Design review of the part built by this model. Coordinates are the model's own, in mm. A direction names the side the tool comes from. Round coordinates to 2 decimals unless told otherwise and drop trailing zeros. Write item = value, one per line.
Autodesk Inventor part; units mm, degrees
ref_plane "Start Plane" through (0, 0, 15) normal (0, 0, 1) x (1, 0, 0)
ref_plane "End Plane" through (0, 0, 435) normal (0, 0, 1) x (1, 0, 0)
ref_plane "Work Plane5" through (-185, 5.2, 435) normal (0, 0, 1) x (1, 0, 0)
ref_plane "Work Plane3" through (0, 0, 250) normal (0, 0, 1) x (1, 0, 0)
sketch "Sketch2" plane through (0, 0, 250) normal (0, 0, 1) x (1, 0, 0)
  circle A0 centre (0, 0) radius 3.4
  dimension "d51" = 6.8
extrude "Extrusion2" [suppressed]
ref_plane "Start Plane" through (0, 0, 15) normal (0, 0, 1) x (1, 0, 0)
ref_plane "End Plane" through (0, 0, 435) normal (0, 0, 1) x (1, 0, 0)
sketch "Sketch" plane through (0, 0, 0) normal (0, 0, 1) x (1, 0, 0)
  line L0 (-13, 15) -> (13, 15)
  line L1 (15, 13) -> (15, -13)
  line L2 (-15, 15) -> (15, -15) construction
  line L3 (15, 15) -> (-15, -15) construction
  line L4 (-5.2, 15) -> (-5.2, 14.2)
  line L5 (-5.2, 14.2) -> (-4.1, 14.2)
  line L6 (-4.1, 14.2) -> (-4.1, 12.2)
  line L7 (-4.1, 12.2) -> (-8.25, 12.2)
  line L8 (-8.25, 12.2) -> (-8.25, 10.2)
  line L9 (-8.25, 10.2) -> (-3.85, 5.8)
  line L10 (-3.85, 5.8) -> (3.85, 5.8)
  line L11 (8.25, 12.2) -> (4.1, 12.2)
  line L12 (4.1, 12.2) -> (4.1, 14.2)
  line L13 (4.1, 14.2) -> (5.2, 14.2)
  line L14 (5.2, 14.2) -> (5.2, 15)
  line L15 (8.25, 12.2) -> (8.25, 10.2)
  line L16 (8.25, 10.2) -> (3.85, 5.8)
  line L17 (-5.8, 0) -> (5.8, 0)
  line L18 (-5.2, -15) -> (-5.2, -14.2)
  line L19 (-5.2, -14.2) -> (-4.1, -14.2)
  line L20 (-4.1, -14.2) -> (-4.1, -12.2)
  line L21 (-4.1, -12.2) -> (-8.25, -12.2)
  line L22 (-8.25, -12.2) -> (-8.25, -10.2)
  line L23 (-8.25, -10.2) -> (-3.85, -5.8)
  line L24 (-3.85, -5.8) -> (3.85, -5.8)
  line L25 (8.25, -12.2) -> (4.1, -12.2)
  line L26 (4.1, -12.2) -> (4.1, -14.2)
  line L27 (4.1, -14.2) -> (5.2, -14.2)
  line L28 (5.2, -14.2) -> (5.2, -15)
  line L29 (8.25, -12.2) -> (8.25, -10.2)
  line L30 (8.25, -10.2) -> (3.85, -5.8)
  line L31 (0, 5.8) -> (0, -5.8)
  line L32 (15, 5.2) -> (14.2, 5.2)
  line L33 (14.2, 5.2) -> (14.2, 4.1)
  line L34 (14.2, 4.1) -> (12.2, 4.1)
  line L35 (12.2, 4.1) -> (12.2, 8.25)
  line L36 (15, -5.2) -> (14.2, -5.2)
  line L37 (14.2, -5.2) -> (14.2, -4.1)
  line L38 (14.2, -4.1) -> (12.2, -4.1)
  line L39 (12.2, -4.1) -> (12.2, -8.25)
  line L40 (12.2, -8.25) -> (10.2, -8.25)
  line L41 (10.2, -8.25) -> (5.8, -3.85)
  line L42 (5.8, -3.85) -> (5.8, 3.85)
  line L43 (5.8, 3.85) -> (10.2, 8.25)
  line L44 (10.2, 8.25) -> (12.2, 8.25)
  line L45 (-15, 5.2) -> (-14.2, 5.2)
  line L46 (-14.2, 5.2) -> (-14.2, 4.1)
  line L47 (-14.2, 4.1) -> (-12.2, 4.1)
  line L48 (-12.2, 4.1) -> (-12.2, 8.25)
  line L49 (-15, -5.2) -> (-14.2, -5.2)
  line L50 (-14.2, -5.2) -> (-14.2, -4.1)
  line L51 (-14.2, -4.1) -> (-12.2, -4.1)
  line L52 (-12.2, -4.1) -> (-12.2, -8.25)
  line L53 (-12.2, -8.25) -> (-10.2, -8.25)
  line L54 (-10.2, -8.25) -> (-5.8, -3.85)
  line L55 (-5.8, -3.85) -> (-5.8, 3.85)
  line L56 (-5.8, 3.85) -> (-10.2, 8.25)
  line L57 (-10.2, 8.25) -> (-12.2, 8.25)
  circle A0 centre (11.5, 11.5) radius 1.65
  circle A1 centre (11.5, -11.5) radius 1.65
  circle A2 centre (-11.5, 11.5) radius 1.65
  circle A3 centre (-11.5, -11.5) radius 1.65
  line L58 (-15, -13) -> (-15, -5.2)
  line L59 (-15, 5.2) -> (-15, 13)
  line L60 (13, -15) -> (5.2, -15)
  line L61 (-5.2, -15) -> (-13, -15)
  arc A4 (-13, 15) -> (-15, 13) centre (-13, 13) ccw
  arc A5 (15, 13) -> (13, 15) centre (13, 13) ccw
  arc A6 (13, -15) -> (15, -13) centre (13, -13) ccw
  arc A7 (-15, -13) -> (-13, -15) centre (-13, -13) ccw
  point P0 (0, 0)
  point P1 (0, 0)
  dimension "d2" = 8.2
  dimension "d3" = 4.1
  dimension "d4" = 10.4
  dimension "d5" = 5.2
  dimension "d8" = 9.2
  dimension "d11" = 16.5
  dimension "d12" = 8.25
  dimension "d14" = 0.8
  dimension "d15" = 2
  dimension "d16" = 2
  dimension "d34" = 0.8
  dimension "d35" = 10.4
  dimension "d36" = 5.2
  dimension "d37" = 8.2
  dimension "d38" = 4.1
  dimension "d39" = 2
  dimension "d40" = 16.5
  dimension "d41" = 8.25
  dimension "d42" = 2
  dimension "d43" = 9.2
  dimension "d44" = 23
  dimension "d45" = 11.5
  dimension "d46" = 23
  dimension "d47" = 11.5
  dimension "d48" = 3.3
  dimension "d55" = 2
extrude "Body" add sketch "Sketch" along normal up to surface (420 mm away) from surface at 15 contours L0 L4 L5 L6 L7 L8 L9 L10 L31 L17 L55 L56 L57 L48 L47 L46 L45 L59 A4 | L0 A5 L1 L32 L33 L34 L35 L44 L43 L42 L17 L31 L10 L16 L15 L11 L12 L13 L14 | L1 A6 L60 L28 L27 L26 L25 L29 L30 L24 L31 L17 L42 L41 L40 L39 L38 L37 L36 | L31 L24 L23 L22 L21 L20 L19 L18 L61 A7 L58 L49 L50 L51 L52 L53 L54 L55 L17
sketch "Sketch3" plane through (0, 0, 0) normal (0, 0, 1) x (1, 0, 0)
  line L0 (0, 0) -> (10, 0)
ref_plane "Work Plane4" through (0, 0, 0) normal (0, -1, 0) x (1, 0, 0)
sketch "Sketch4" plane through (0, 0, 0) normal (0, -1, 0) x (1, 0, 0)
  line L0 (-2, 15) -> (12, 15)
  line L1 (-2, 435) -> (12, 435)
  dimension "d61" = 420
ref_plane "Work Plane5" through (-185, 5.2, 435) normal (0, 0, 1) x (1, 0, 0)
split "Split1" plane through (-185, 5.2, 435) removes the side toward (0, 0, 1)
ref_plane "Work Plane6" through (265, 5.2, 15) normal (0, 0, -1) x (-1, 0, 0)
split "Split2" plane through (265, 5.2, 15) removes the side toward (0, 0, -1)
equation "\"d3\" = 0.5 * d2"
equation "\"G_OFFSET_START\" = -15"
equation "\"G_OFFSET_END\" = -15"
equation "\"d56\" = -G_OFFSET_START"
equation "\"G_L\" = d61"
properties part number "420 mm" material "Aluminum 6061"
Item 1: Take a section at A-A, the plane z = 128.5. Count the separate pieces of the cut face and the enclosed holes in it, and give its area (3 significant figures).
Data:
separate_pieces = 1
enclosed_holes = 4
area = 419 mm2
Item 2: Insertion check: P1, Ø2, axis at x = 11.5, y = 11.5, coming from the -Z side; P2, Ø1, axis at y = 1.5, z = 273.5, coming from the -X side; P3, Ø5, axis at x = 0.5, z = 115.5, coming from the +Y side; P4, Ø0.9, axis at x = -4.5, z = 121, coming from the +Y side. Each pin has a flat end and moves straight along its axis. Give the tip position at first contact, or say it passes through.
Data:
P1 = through
P2 = -5.8
P3 = 5.8
P4 = 14.2
Item 3: For faces 4 (the face through (-5.8, 0, 222)), 5 (the face through (0, -5.8, 222)), 6 (the face through (5.8, 0, 222)), list the 3-axis set-ups (+Z, -Z, +X, -X, +Y, -Y) from which the entire face can be reached by the end or side of a thin tool; tool diameter is ignored.
Data:
face_4 = +Z, -Z, -X
face_5 = +Z, -Z, -Y
face_6 = +Z, -Z, +X
Item 4: For line 1 along Y through (x, z) = (-11.5, 205.5); line 2 along X through (y, z) = (-12, 313.5); line 3 along X through (y, z) = (-4.5, 226.5), list the stretches that pass through material, from the lowest coordinate up. Write a range as [from, to].
Data:
line_1 = [-15, -13.15], [-9.85, -8.25], [8.25, 9.85], [13.15, 15]
line_2 = [-15, -13.07], [-9.93, -8.25], [8.25, 9.93], [13.07, 15]
line_3 = [-14.2, -12.2], [-6.45, 6.45], [12.2, 14.2]
Item 5: The part is to be moulded in two halves that separate along X. For faces 1 (the face through (0, 5.8, 222)), 2 (the face through (0, 0, 435)), 3 (the face through (-15, 9, 222)), say which applies: +X half, -X half, draft (parallel to the pull), parting line (faces both ways), or undercut.
Data:
face_1 = undercut
face_2 = draft
face_3 = -X half
